from build123d import *

# Parameters (mm, degrees)
SKETCH1_R           = 17.5
BOSS_EXTRUDE1_DEPTH = 1
SKETCH2_R           = 4
CUT_EXTRUDE1_DEPTH  = 5


with BuildPart() as part:
    # Sketch1 → Boss-Extrude1 (new body)
    with BuildSketch(Plane(origin=(0, 0, 0), x_dir=(1, 0, 0), z_dir=(0, 1, 0))):
        with Locations(Location((0, 0, 0), (0, 0, 270))):
            Circle(SKETCH1_R)
        with BuildLine():
            Line((14.66, 1.27), (12.12, 1.27))
            ThreePointArc((12.12, 1.27), (10.85, 0), (12.12, -1.27))
            Line((12.12, -1.27), (14.66, -1.27))
            ThreePointArc((14.66, -1.27), (15.93, 0), (14.66, 1.27))
        make_face(mode=Mode.SUBTRACT)
        with BuildLine():
            Line((-14.66, -1.27), (-12.12, -1.27))
            ThreePointArc((-12.12, -1.27), (-10.85, 0), (-12.12, 1.27))
            Line((-12.12, 1.27), (-14.66, 1.27))
            ThreePointArc((-14.66, 1.27), (-15.93, 0), (-14.66, -1.27))
        make_face(mode=Mode.SUBTRACT)
    extrude(amount=BOSS_EXTRUDE1_DEPTH)

    # Sketch2 → Cut-Extrude1 (cut, symmetric)
    with BuildSketch(Plane(origin=(0, 1, 0), x_dir=(1, 0, 0), z_dir=(0, 1, 0))):
        with Locations(Location((0, 0, 0), (0, 0, 270))):
            Circle(SKETCH2_R)
    extrude(amount=CUT_EXTRUDE1_DEPTH, both=True, mode=Mode.SUBTRACT)


solid = part.part
Build history of the part. All positions in model axes, mm. A direction names the side the tool comes from. Coordinates: 2 decimals unless noted, no trailing zeros. Order: outer loops, then holes, each group sorted by start corner. A loop starts at its lowest first (then second) coordinate and runs counter-clockwise, first axis right, second up. Notation, with made-up numbers: (88, -16) - (118, -16) arc R25 ccw to (118, 22) - close; hole circle Ø1 at (-22.5, 23). An arc over 180 degrees is marked (long way). Write item = value, one per line. Start each with the question number.
1) Flat gauge pins, fed straight in: pin 1 Ø0.5 at (x, y) = (13, 0.5) entering from +Z; pin 2 Ø10 at (x, z) = (-11, -14) entering from +Y. Where does each tip first touch, or does it go through?
2) Two-plate mould, pull along Z, no slides. Class faces 3 (the face through (-10.648, 0.493, -13.887)), 4 (the face through (10.85, 0.49, -0.03)), 5 (the face through (-4, 0, 4)): pulls with the +Z half, pulls with the -Z half, needs draft (parallel to the pull), parting line crosses it, or undercut.
3) Saw through at C-C on x = 0. Write the cut outline in (y, z), then the cut area to 3 significant figures.
4) Wall check: line 1 along X through (y, z) = (0.45, 0); line 2 along X through (y, z) = (0.85, 0.5); line 3 along Z through (x, y) = (-15.5, 0.2). Give the ranges that are in metal, low to high. Write a range as from..to.
5) Saw through at B-B on y = 0.3. Write the cut outline in (x, z).
6) Saw through at D-D on x = -11.5. Write the cut outline in (y, z).
7) Saw through at A-A on z = 0. Write the cut outline in (x, y).
8) 3-axis set-ups, long thin cutter, end or side, ignore diameter. For faces 1 (the face through (13.4, 0.5, -1.27)), 2 (the face through (-4, 1, 4)): which of +Z, -Z, +X, -X, +Y, -Y reach the whole face in a straight line?
From the geometry:
q1.pin_1 = 11.99
q1.pin_2 = 1
q2.face_3 = parting line crosses it
q2.face_4 = undercut
q2.face_5 = needs draft
q3.outline = (0, -17.5) - (1, -17.5) - (1, -4) - (0, -4) - close; (0, 4) - (1, 4) - (1, 17.5) - (0, 17.5) - close
q3.area = 27.0 mm^2
q4.line_1 = -17.5..-15.93, -10.85..-4, 4..10.85, 15.93..17.5
q4.line_2 = -17.49..-15.83, -10.95..-3.97, 3.97..10.95, 15.83..17.49
q4.line_3 = -8.12..-0.95, 0.95..8.12
q5.outline = circle Ø35 at (0, 0); hole (-14.66, -1.27) - (-12.12, -1.27) arc R1.27 ccw to (-12.12, 1.27) - (-14.66, 1.27) arc R1.27 ccw to start; hole circle Ø8 at (0, 0); hole (12.12, -1.27) - (14.66, -1.27) arc R1.27 ccw to (14.66, 1.27) - (12.12, 1.27) arc R1.27 ccw to start
q6.outline = (0, -13.19) - (1, -13.19) - (1, -1.11) - (0, -1.11) - close; (0, 1.11) - (1, 1.11) - (1, 13.19) - (0, 13.19) - close
q7.outline = (-17.5, 0) - (-15.93, 0) - (-15.93, 1) - (-17.5, 1) - close; (-10.85, 0) - (-4, 0) - (-4, 1) - (-10.85, 1) - close; (4, 0) - (10.85, 0) - (10.85, 1) - (4, 1) - close; (15.93, 0) - (17.5, 0) - (17.5, 1) - (15.93, 1) - close
q8.face_1 = +Y, -Y
q8.face_2 = +Z, -Z, +X, -X, +Y
